```python
from build123d import *

# Parameters (mm, degrees)
SKETCH1_R           = 2.000000064
BOSS_EXTRUDE1_DEPTH = 61.9125


with BuildPart() as part:
    # Sketch1 → Boss-Extrude1 (new, symmetric)
    with BuildSketch(Plane.XY):
        with BuildLine():
            ThreePointArc((4.181770846, 5.456960429), (3.437499983, 5.953924622), (2.634980936, 6.35))
            Line((2.634980936, 6.35), (-2.634980936, 6.35))
            ThreePointArc((-2.634980936, 6.35), (-3.437499983, 5.953924622), (-4.181770846, 5.456960429))
            Line((-4.181770846, 5.456960429), (-6.816751782, 0.893039571))
            ThreePointArc((-6.816751782, 0.893039571), (-6.874999966, 0), (-6.816751782, -0.893039571))
            Line((-6.816751782, -0.893039571), (-4.181770846, -5.456960429))
            ThreePointArc((-4.181770846, -5.456960429), (-3.437499983, -5.953924622), (-2.634980936, -6.35))
            Line((-2.634980936, -6.35), (2.634980936, -6.35))
            ThreePointArc((2.634980936, -6.35), (3.437499983, -5.953924622), (4.181770846, -5.456960429))
            Line((4.181770846, -5.456960429), (6.816751782, -0.893039571))
            ThreePointArc((6.816751782, -0.893039571), (6.860422465, -0.447468582), (6.874999966, 0))
            ThreePointArc((6.874999966, 0), (6.860422465, 0.447468582), (6.816751782, 0.893039571))
            Line((6.816751782, 0.893039571), (4.181770846, 5.456960429))
        make_face()
        Circle(SKETCH1_R, mode=Mode.SUBTRACT)
    extrude(amount=BOSS_EXTRUDE1_DEPTH, both=True)


solid = part.part
```
Geometry check sheet. Reference: the model listing, model coordinates, mm. Give positions to 0.01 mm unless a question says otherwise; leave off trailing zeros. Write each loop counter-clockwise with the first axis right and the second up, starting at its lowest first coordinate (ties: lowest second). Pieces come first, ordered by that corner, then holes.
1) Section check B-B, the plane z = -9. Record the boundary of the cut face in (x, y) (3 decimals).
2) Section check A-A, the plane x = 0. Record the boundary of the cut face in (y, z).
3) Gauge pin test, flat ends, axial feed: pin 1 (5 mm diameter, centred on y = 1.5, z = -41.5, fed in from -X) (3 decimals); pin 2 (3 mm diameter, centred on y = 2.5, z = -40.5, fed in from +X) (3 decimals). Record the tip position at first contact, or that the pin passes through.
4) Material ranges on L1, parallel to Y at x = 0, z = 13.5; L2, parallel to Y at x = -1.25, z = 22.5; L3, parallel to X at y = 1.5, z = 18.5, recorded low to high.
Computed:
1. outline: (-6.817, -0.893) - (-4.182, -5.457) arc R6.875 ccw to (-2.635, -6.35) - (2.635, -6.35) arc R6.875 ccw to (4.182, -5.457) - (6.817, -0.893) arc R6.875 ccw to (6.817, 0.893) - (4.182, 5.457) arc R6.875 ccw to (2.635, 6.35) - (-2.635, 6.35) arc R6.875 ccw to (-4.182, 5.457) - (-6.817, 0.893) arc R6.875 ccw to start; hole circle Ø4 at (0, 0)
2. outline: (-6.35, -61.91) - (-2, -61.91) - (-2, 61.91) - (-6.35, 61.91) - close; (2, -61.91) - (6.35, -61.91) - (6.35, 61.91) - (2, 61.91) - close
3. pin 1: stops at x = -6.875
3. pin 2: stops at x = 6.755
4. L1: y = -6.35 to -2, 2 to 6.35
4. L2: y = -6.35 to -1.56, 1.56 to 6.35
4. L3: x = -6.47 to -1.32, 1.32 to 6.47
